from build123d import *

# Parameters (mm, degrees)
BOSS_EXTRUDE1_DEPTH        = 1
F_4_3_4_3_DIAMETER_HOLE1_D = 4.3
SKETCH6_W                  = 28.17
SKETCH6_H                  = 2.5
BOSS_EXTRUDE2_DEPTH        = 23.53


with BuildPart() as part:
    # Sketch1 → Revolve1 (revolve)
    with BuildSketch(Plane(origin=(0, 0, 0), x_dir=(0, 0, -1), z_dir=(1, 0, 0)), mode=Mode.PRIVATE) as revolve1_sk:
        Polygon((60.11, 0), (60.11, 18), (35.01, 18), (35.01, 30.085), (24.6, 30.085), (24.6, 35.25), (5.83, 38.44), (5.83, 44.25), (4.83, 44.25), (4.83, 36.5), (0, 36.5), (0, 0), align=None)
    revolve(revolve1_sk.sketch.rotate(Axis((0, 0, 0), (0, 0, -1)), 90), axis=Axis((0, 0, 0), (0, 0, -1)))

    # Sketch2 → Boss-Extrude1 (add)
    with BuildSketch(Plane.XY.offset(-4.83)):
        with BuildLine():
            ThreePointArc((-35.456787888, 37.168658693), (0, 44.25), (35.456787888, 37.168658693))
            ThreePointArc((35.456787888, 37.168658693), (36.482290492, 36.482290492), (37.168658693, 35.456787888))
            ThreePointArc((37.168658693, 35.456787888), (44.25, 0), (37.168658693, -35.456787888))
            ThreePointArc((37.168658693, -35.456787888), (36.482290492, -36.482290492), (35.456787888, -37.168658693))
            ThreePointArc((35.456787888, -37.168658693), (0, -44.25), (-35.456787888, -37.168658693))
            ThreePointArc((-35.456787888, -37.168658693), (-36.482290492, -36.482290492), (-37.168658693, -35.456787888))
            ThreePointArc((-37.168658693, -35.456787888), (-44.25, 0), (-37.168658693, 35.456787888))
            ThreePointArc((-37.168658693, 35.456787888), (-36.482290492, 36.482290492), (-35.456787888, 37.168658693))
        make_face()
    extrude(amount=-BOSS_EXTRUDE1_DEPTH)

    # Ø4.3 (4.3) Diameter Hole1 (through all)
    with Locations(Plane.XY.offset(-4.83)):
        with Locations((-32.880465325, 32.880465325), (32.880465325, 32.880465325), (32.880465325, -32.880465325), (-32.880465325, -32.880465325)):
            Hole(F_4_3_4_3_DIAMETER_HOLE1_D / 2)

    # Sketch6 → Boss-Extrude2 (add)
    with BuildSketch(Plane(origin=(0, 0, -5.83), x_dir=(-1, 0, 0), z_dir=(0, 0, -1))):
        with Locations((0, -38.6)):
            Rectangle(SKETCH6_W, SKETCH6_H)
    extrude(amount=BOSS_EXTRUDE2_DEPTH)


solid = part.part
The listing builds one solid part. Answer for the finished solid, in the listing's coordinates (mm). A direction names the side the tool comes from. Coordinates: 2 decimals unless noted, no trailing zeros. Write each loop counter-clockwise with the first axis right and the second up, starting at its lowest first coordinate (ties: lowest second). Pieces come first, ordered by that corner, then holes. Notation, with made-up numbers: (-18, 73.5) - (11, 73.5) arc R9 ccw to (11, 84.5) - close; hole circle Ø3 at (48, -21.5). An arc over 180 degrees is marked (long way). Put each result on its own line as item: value.
1. The part is cut by section C-C on x = -33. State how many separate pieces and enclosed holes the cut face has, plus the area to 3 significant figures.
Answer sheet:
separate pieces: 3
enclosed holes: 0
area: 829 mm^2
2. The part is cut by section A-A on z = -18.5. Give the vertices of the cut face in (x, y) (3 decimals), plus the area to 3 significant figures.
Answer sheet:
outline: circle Ø72.573 at (0, 0); (-14.085, -39.85) - (14.085, -39.85) - (14.085, -37.35) - (-14.085, -37.35) - close
area: 4,210 mm^2
3. The part is cut by section D-D on z = -26.5. Give the vertices of the cut face in (x, y) (3 decimals).
Answer sheet:
outline: circle Ø60.17 at (0, 0); (-14.085, -39.85) - (14.085, -39.85) - (14.085, -37.35) - (-14.085, -37.35) - close
4. Flat-ended cylindrical pins translate along their axes: pin 1 Ø10 at (y, z) = (12.5, -31.5) entering from +X; pin 2 Ø5.5 at (x, y) = (32.88, -32.88) entering from -Z; pin 3 Ø3 at (y, z) = (-38.5, -20.5) entering from -X (3 decimals). Find the tip coordinate at first contact, or state that the pin passes through.
Answer sheet:
pin 1: stops at x = 29.14
pin 2: stops at z = -5.83
pin 3: stops at x = -14.085
5. Find the intervals of material crossed by line 1 along Z through (x, y) = (30, -30.5); line 2 along Z through (x, y) = (27, 2); line 3 along Y through (x, z) = (-10.5, -28.5), in increasing order. Write a range as from..to.
Answer sheet:
line 1: z = -5.83..-4.83
line 2: z = -35.01..0
line 3: y = -39.85..-37.35, -28.19..28.19
6. A tool of negligible diameter and unlimited length cuts with its end or side. For faces 5 (the face through (16.843, 32.382, -2.381)), 6 (the face through (0, -39, -29.36)), 7 (the face through (-14.085, -39, -17)), 8 (the face through (-13.267, -12.165, -47.384)), from which of +Z, -Z, +X, -X, +Y, -Y can it reach the whole face along a straight path? Write none if from no direction.
Answer sheet:
face 5: +Z
face 6: -Z, +X, -X, -Y
face 7: -Z, -X, -Y
face 8: -Z
7. Determine the mould class of faces 1 (the face through (-30.733, -32.786, -5.337)), 2 (the face through (-0.51, 44.25, -5.32)), 3 (the face through (-44.25, -0.51, -5.32)), 4 (the face through (-1, -1, 0)) for opening direction X: pulls with the +X half, pulls with the -X half, needs draft (parallel to the pull), parting line crosses it, or undercut.
Answer sheet:
face 1: undercut
face 2: parting line crosses it
face 3: pulls with the -X half
face 4: needs draft
8. The part is cut by section B-B on y = 0. Give the vertices of the cut face in (x, z) (3 decimals).
Answer sheet:
outline: (-44.25, -5.83) - (-38.44, -5.83) - (-35.25, -24.6) - (-30.085, -24.6) - (-30.085, -35.01) - (-18, -35.01) - (-18, -60.11) - (18, -60.11) - (18, -35.01) - (30.085, -35.01) - (30.085, -24.6) - (35.25, -24.6) - (38.44, -5.83) - (44.25, -5.83) - (44.25, -4.83) - (36.5, -4.83) - (36.5, 0) - (-36.5, 0) - (-36.5, -4.83) - (-44.25, -4.83) - close
